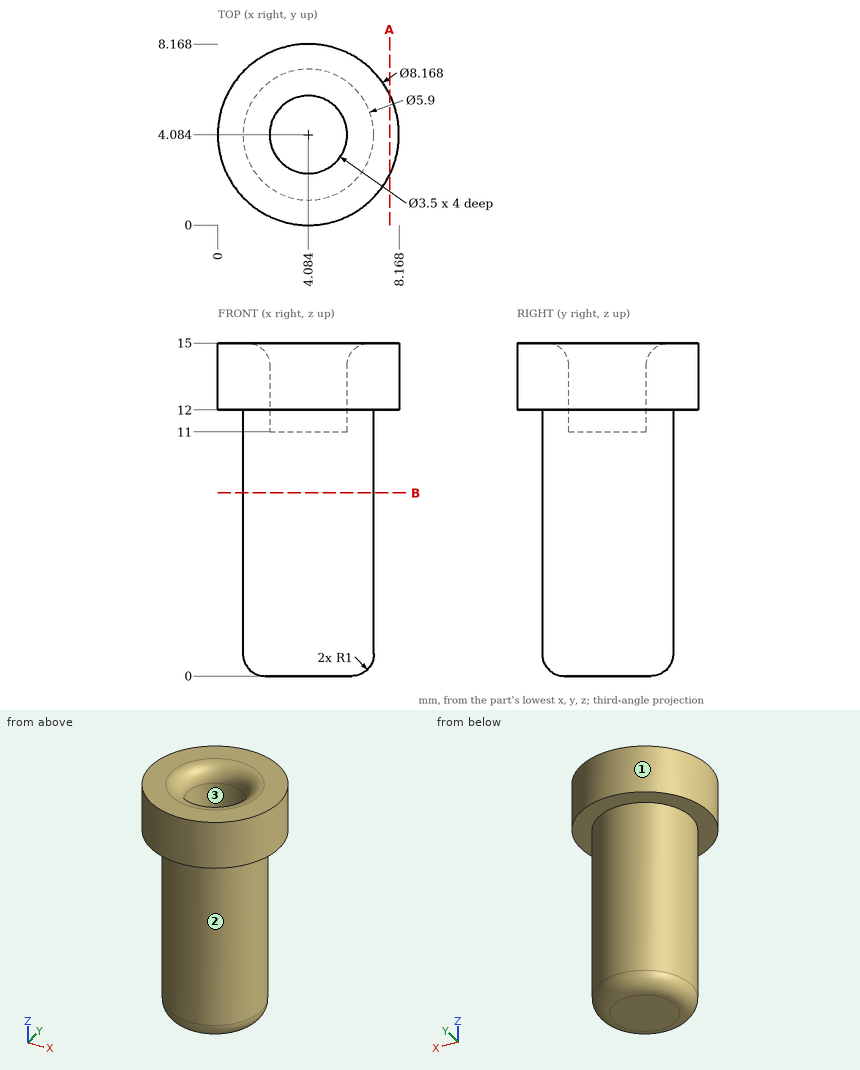
Here's the drawing with two shaded views (mm, measured from the low corner). I have some questions. A direction names the side the tool comes from. Coordinates: 2 decimals unless noted, no trailing zeros. Write each loop counter-clockwise with the first axis right and the second up, starting at its lowest first coordinate (ties: lowest second). Pieces come first, ordered by that corner, then holes. Notation, with made-up numbers: (-36.75, 19) -> (-3.75, 19) arc R13 ccw to (-3.75, 31) -> close; hole circle Ø2 at (48.25, 84.5). An arc over 180 degrees is marked (long way). One line per question, with ' | ' between items. Start each with the question number.
1. Please list where these lines run through material, in increasing order: line 1 along Y through (x, z) = (5.25, 13.25); line 2 along Y through (x, z) = (2.5, 13.5); line 3 along Z through (x, y) = (1.5, 2).
2. If we section it at B-B (z = 8.25): Please give me the cut outline in (x, y), and give its area (3 significant figures).
3. Will these pins go through, and if not, where does the flat tip stop? P1, Ø1.5, axis at y = 4, z = 4, coming from the +X side; P2, Ø4, axis at x = 3.5, y = 4, coming from the +Z side; P3, Ø3, axis at x = 3, z = 7, coming from the +Y side; P4, Ø3, axis at x = 5.5, z = 11.5, coming from the +Y side.
4. For the marked faces 1, 2 and 3, which set-ups out of +Z, -Z, +X, -X, +Y, -Y let a thin tool reach every point of the face, with its end or its side?
5. If we section it at A-A (x = 7.75): Please give me the cut outline in (y, z).
Return value:
1) line 1: y = 0.17 to 2.78, 5.39 to 8 | line 2: y = 0.32 to 3.34, 4.83 to 7.85 | line 3: z = 12 to 15
2) outline: circle Ø5.9 at (4.08, 4.08) | area: 27.3 mm²
3) P1: stops at x = 7.03 | P2: stops at z = 14.99 | P3: stops at y = 7.03 | P4: stops at y = 8.17
4) face 1: +Z, -Z | face 2: -Z | face 3: +Z
5) outline: (2.28, 12) -> (5.88, 12) -> (5.88, 15) -> (2.28, 15) -> close
